Design review of the part built by this model. Coordinates are the model's own, in mm. A direction names the side the tool comes from. Give positions to 0.01 mm unless a question says otherwise; leave off trailing zeros. Write each loop counter-clockwise with the first axis right and the second up, starting at its lowest first coordinate (ties: lowest second). Pieces come first, ordered by that corner, then holes. Notation, with made-up numbers: M 33.25,37.5 L 92.25,37.5 A22 cw 92.25,43.5 Z; hole C -40,78 d11. An arc over 180 degrees is marked long. Answer in a Markdown table with one row per item.
```python
from build123d import *

# Parameters (mm, degrees)
BOSS_EXTRUDE1_DEPTH = 2.54
SKETCH2_R           = 47.6885
BOSS_EXTRUDE2_DEPTH = 2.54
SKETCH3_R           = 4.7625
CUT_EXTRUDE1_DEPTH  = 5.08
BOSS_EXTRUDE4_DEPTH = 19.05


with BuildPart() as part:
    # Sketch1 → Boss-Extrude1 (new body)
    with BuildSketch(Plane(origin=(0, 0, 0), x_dir=(1, 0, 0), z_dir=(0, 1, 0))):
        with BuildLine():
            Line((-49.5046, 0), (-47.6885, 0))
            ThreePointArc((-47.6885, 0), (0, -47.6885), (47.6885, 0))
            Line((47.6885, 0), (49.5046, 0))
            ThreePointArc((49.5046, 0), (0, 49.5046), (-49.5046, 0))
        make_face()
    extrude(amount=BOSS_EXTRUDE1_DEPTH)

    # Sketch2 → Boss-Extrude2 (add)
    with BuildSketch(Plane(origin=(0, 2.54, 0), x_dir=(1, 0, 0), z_dir=(0, 1, 0))):
        Circle(SKETCH2_R)
    extrude(amount=BOSS_EXTRUDE2_DEPTH)

    # Sketch3 → Cut-Extrude1 (cut)
    with BuildSketch(Plane.XZ):
        with Locations(Location((12.7, 31.235352443, 0), (0, 0, 270))):
            Circle(SKETCH3_R)
        with Locations(Location((-12.7, 31.235352443, 0), (0, 0, 270))):
            Circle(SKETCH3_R)
    extrude(amount=-CUT_EXTRUDE1_DEPTH, mode=Mode.SUBTRACT)

    # Sketch4 → Boss-Extrude4 (add)
    with BuildSketch(Plane.XZ):
        Polygon((41.959363096, 22.662852443), (-41.959363096, 22.662852443), (-39.665868398, 26.472852443), (39.665868398, 26.472852443), align=None)
    extrude(amount=BOSS_EXTRUDE4_DEPTH)


solid = part.part
```
1) Add section C-C (y = -10.75). Write out the cut boundary in (x, z).
Geometry says:
| item | result |
|---|---|
| outline | M -41.96,22.66 L 41.96,22.66 L 39.67,26.47 L -39.67,26.47 Z |
2) Add section A-A (x = 0). Write out the cut boundary in (y, z).
Geometry says:
| item | result |
|---|---|
| outline | M -19.05,22.66 L 0,22.66 L 0,-49.5 L 2.54,-49.5 L 2.54,-47.69 L 5.08,-47.69 L 5.08,47.69 L 0,47.69 L 0,26.47 L -19.05,26.47 Z |
3) For faces 1 (the face through (22.005, 3.069, 42.308)), 2 (the face through (-1, 0, 37)), 3 (the face through (-11.269, 2.504, 26.693)), 4 (the face through (-1, 0, -6)), 5 (the face through (0, 2.54, -49)), list the 3-axis set-ups (+Z, -Z, +X, -X, +Y, -Y) from which the entire face can be reached by the end or side of a thin tool; tool diameter is ignored.
Geometry says:
| item | result |
|---|---|
| face 1 | +Y |
| face 2 | +Z, +X, -X, -Y |
| face 3 | +Y, -Y |
| face 4 | -Z, +X, -X, -Y |
| face 5 | -Z, +Y |
4) To check wall thickness, follow probe 1 along Z at (x, y) = (6.5, -4.75); probe 2 along Y at (x, z) = (-4.5, 4); probe 3 along Z at (x, y) = (-9, 1). State the ranges of each line that lie inside material, in increasing order. Write a range as [from, to].
Geometry says:
| item | result |
|---|---|
| probe 1 | [22.66, 26.47] |
| probe 2 | [0, 5.08] |
| probe 3 | [-48.68, 28.24], [34.23, 46.83] |
5) Insertion check: P1, Ø6, axis at x = -7, z = 17, coming from the -Y side; P2, Ø3, axis at x = 3, y = -16, coming from the -Z side; P3, Ø8, axis at x = 26.5, y = -8.5, coming from the +Z side; P4, Ø8.5, axis at x = 12.7, z = 31.24, coming from the +Y side. Each pin has a flat end and moves straight along its axis. Give the tip position at first contact, or say it passes through.
Geometry says:
| item | result |
|---|---|
| P1 | y = 0 |
| P2 | z = 22.66 |
| P3 | z = 26.47 |
| P4 | through |
6) Add section D-D (z = 15.5). Write out the cut boundary in (x, y).
Geometry says:
| item | result |
|---|---|
| outline | M -45.1,0 L 45.1,0 L 45.1,5.08 L -45.1,5.08 Z |
7) Add section B-B (x = -14.5). Write out the cut boundary in (y, z).
Geometry says:
| item | result |
|---|---|
| outline | M -19.05,22.66 L 0,22.66 L 0,-47.33 L 2.54,-47.33 L 2.54,-45.43 L 5.08,-45.43 L 5.08,26.83 L 0,26.83 L 0,26.47 L -19.05,26.47 Z; M 0,35.64 L 5.08,35.64 L 5.08,45.43 L 0,45.43 Z |
